from build123d import *

# Parameters (mm, degrees)
BOSS_EXTRUDE2_DEPTH = 20
SKETCH3_R           = 5.75
CUT_EXTRUDE1_DEPTH  = 21


with BuildPart() as part:
    # Sketch2 → Boss-Extrude2 (new body)
    with BuildSketch(Plane(origin=(0, 0, 0), x_dir=(1, 0, 0), z_dir=(0, 1, 0))):
        Polygon((-12.666179626, 10), (-12.666179626, -15), (164.478056179, -263.93698429), (164.478056179, -283.967221838), (189.810415431, -283.967221838), (189.810415431, -263.93698429), (12.666179626, -15), (12.666179626, 10), align=None)
    extrude(amount=BOSS_EXTRUDE2_DEPTH)

    # Sketch3 → Cut-Extrude1 (cut, through all)
    with BuildSketch(Plane(origin=(0, 20, 0), x_dir=(1, 0, 0), z_dir=(0, 1, 0))):
        Circle(SKETCH3_R)
        with Locations((182.478056179, -276.967221838)):
            Circle(SKETCH3_R)
    extrude(amount=-CUT_EXTRUDE1_DEPTH, mode=Mode.SUBTRACT)


solid = part.part
Could you check a few things on this model? Use its own coordinates, in mm. A direction names the side the tool comes from. Coordinates: 2 decimals unless noted, no trailing zeros. Order: outer loops, then holes, each group sorted by start corner. A loop starts at its lowest first (then second) coordinate and runs counter-clockwise, first axis right, second up.
Q1. Suppose I cut it at C-C on y = 3.25. Please give me the cut outline in (x, z), and give its area (3 significant figures).
Q2. Which directions (+Z, -Z, +X, -X, +Y, -Y) give clear straight access to the entire face, cutting with the end or side of a thin tool? Please do faces 4 (the flat face through (164.478, 10, 274)), 5 (the flat face through (12.666, 10, 3)), 6 (the flat face through (-12.666, 10, 2)).
Q3. Suppose I cut it at D-D on x = 77.5. Please give me the cut outline in (y, z), and give its area (3 significant figures).
Q4. Suppose I cut it at B-B on x = 2. Please give me the cut outline in (y, z).
Q5. Please list where these lines run through material, in increasing order: L1, parallel to Z at x = 0, y = 9; L2, parallel to X at y = 13.5, z = 0; L3, parallel to X at y = 17, z = 4.
Q6. Thinking about a two-plate mould opening in Z: for faces 1 (the cylindrical face through (185.13, 10.14, 282.07)), 2 (the flat face through (0, 10, -10)), 3 (the flat face through (81, 0, 125)), which applies, released by +Z, released by -Z, zero draft, split by the parting line, or undercut?
Q7. Will these pins go through, and if not, where does the flat tip stop? pin 1 (3 mm diameter, centred on x = 20.5, y = 16.5, fed in from +Z); pin 2 (12 mm diameter, centred on x = 121.5, y = 15.5, fed in from +Z); pin 3 (12 mm diameter, centred on x = 91.5, y = 5, fed in from -Z).
Q8. Suppose I cut it at A-A on z = 0. Please give me the cut outline in (x, y), and give its area (3 significant figures).
Answer:
1. outline: (-12.67, -10) - (12.67, -10) - (12.67, 15) - (189.81, 263.94) - (189.81, 283.97) - (164.48, 283.97) - (164.48, 263.94) - (-12.67, 15) - close; hole circle Ø11.5 at (0, 0); hole circle Ø11.5 at (182.48, 276.97)
1. area: 7,240 mm2
2. face 4: +Z, -X, +Y, -Y
2. face 5: -Z, +X, +Y, -Y
2. face 6: +Z, -Z, -X, +Y, -Y
3. outline: (0, 106.11) - (20, 106.11) - (20, 141.71) - (0, 141.71) - close
3. area: 712 mm2
4. outline: (0, -10) - (20, -10) - (20, -5.39) - (0, -5.39) - close; (0, 5.39) - (20, 5.39) - (20, 35.61) - (0, 35.61) - close
5. L1: z = -10 to -5.75, 5.75 to 32.8
5. L2: x = -12.67 to -5.75, 5.75 to 12.67
5. L3: x = -12.67 to -4.13, 4.13 to 12.67
6. face 1: undercut
6. face 2: released by -Z
6. face 3: zero draft
7. pin 1: stops at z = 63.72
7. pin 2: stops at z = 211.97
7. pin 3: stops at z = 117.35
8. outline: (-12.67, 0) - (-5.75, 0) - (-5.75, 20) - (-12.67, 20) - close; (5.75, 0) - (12.67, 0) - (12.67, 20) - (5.75, 20) - close
8. area: 277 mm2
